Work out the finished part from the listing and answer in its coordinate system (mm). A direction names the side the tool comes from. Coordinates: 2 decimals unless noted, no trailing zeros. Loops run counter-clockwise (first coordinate to the right, second up) from the corner with the lowest first, then second, coordinate; pieces in that order, holes last. Notation, with made-up numbers: M 26.5,-19.5 L 68.5,-19.5 A19 ccw 68.5,-3.5 Z; hole C 42,81 d6. An arc over 180 degrees is marked long. Write each question's results on one line, items separated by ' | '.
```python
from build123d import *

# Parameters (mm, degrees)
SKETCH1_R           = 10.25
BOSS_EXTRUDE1_DEPTH = 2
SKETCH2_R           = 3.4
SKETCH2_R_2         = 2.9
BOSS_EXTRUDE2_DEPTH = 1
SKETCH3_R           = 1.35
CUT_EXTRUDE1_DEPTH  = 15.633010627
SKETCH4_R           = 0.7
CUT_EXTRUDE2_DEPTH  = 15.633010627
CIRPATTERN1_COUNT   = 4
SKETCH5_R           = 4.85
SKETCH5_R_2         = 2.7
BOSS_EXTRUDE3_DEPTH = 3


with BuildPart() as part:
    # Sketch1 → Boss-Extrude1 (new body)
    with BuildSketch(Plane.XY):
        Circle(SKETCH1_R)
    extrude(amount=BOSS_EXTRUDE1_DEPTH)

    # Sketch2 → Boss-Extrude2 (add)
    with BuildSketch(Plane.XY.offset(2)):
        Circle(SKETCH2_R)
        Circle(SKETCH2_R_2, mode=Mode.SUBTRACT)
    extrude(amount=BOSS_EXTRUDE2_DEPTH)

    # Sketch3 → Cut-Extrude1 (cut, through all)
    with BuildSketch(Plane.XY.offset(2)):
        Circle(SKETCH3_R)
    extrude(amount=-CUT_EXTRUDE1_DEPTH, mode=Mode.SUBTRACT)

    # Sketch4 → Cut-Extrude2 (cut, through all)
    with BuildSketch(Plane.XY.offset(2)):
        with Locations((0, 7.25)):
            Circle(SKETCH4_R)
        with Locations((3.5, 7.25)):
            Circle(SKETCH4_R)
        with Locations(Location((-3.5, 7.25, 0), (0, 0, 180))):
            Circle(SKETCH4_R)
        with Locations((-3.5, -7.25)):
            Circle(SKETCH4_R)
        with Locations(Location((3.5, -7.25, 0), (0, 0, 180))):
            Circle(SKETCH4_R)
        with Locations(Location((0, -7.25, 0), (0, 0, 180))):
            Circle(SKETCH4_R)
    cut_extrude2 = extrude(amount=-CUT_EXTRUDE2_DEPTH, mode=Mode.SUBTRACT)

    # CirPattern1: Cut-Extrude2 ×4 about axis
    cirpattern1_axis = Axis((0, 0, 0), (0, 0, 1))
    for i in range(1, CIRPATTERN1_COUNT):
        add(cut_extrude2.rotate(cirpattern1_axis, i * 360 / CIRPATTERN1_COUNT), mode=Mode.SUBTRACT)

    # Sketch5 → Boss-Extrude3 (add)
    with BuildSketch(Plane(origin=(0, 0, 0), x_dir=(-1, 0, 0), z_dir=(0, 0, -1))):
        with Locations(Location((0, 0, 0), (0, 0, 180))):
            Circle(SKETCH5_R)
        Circle(SKETCH5_R_2, mode=Mode.SUBTRACT)
    extrude(amount=BOSS_EXTRUDE3_DEPTH)


solid = part.part
```
1) Find section C-C, the plane y = -7.25. Give the vertices of the cut face in (x, z).
Check result:
outline: M -7.25,0 L -4.2,0 L -4.2,2 L -7.25,2 Z; M -2.8,0 L -0.7,0 L -0.7,2 L -2.8,2 Z; M 0.7,0 L 2.8,0 L 2.8,2 L 0.7,2 Z; M 4.2,0 L 7.25,0 L 7.25,2 L 4.2,2 Z
2) For a pull along Y with two mould halves and no side action, classify faces 4 (the face through (-2.222, -10.006, 0.986)), 5 (the face through (3, 1, 3)), 6 (the face through (-7.84, 0.38, 1.01)) as released by +Y, released by -Y, zero draft, split by the parting line, or undercut.
Check result:
face 4: split by the parting line | face 5: zero draft | face 6: undercut
3) Find section D-D, the plane y = 3.75. Give the vertices of the cut face in (x, z).
Check result:
outline: M -9.54,0 L -7.9,0 L -7.9,2 L -9.54,2 Z; M -6.6,0 L -3.08,0 L -3.08,-3 L 3.08,-3 L 3.08,0 L 6.6,0 L 6.6,2 L -6.6,2 Z; M 7.9,0 L 9.54,0 L 9.54,2 L 7.9,2 Z
4) Find section A-A, the plane x = 0. Give the number of separate pieces and of enclosed holes in the cut face, and give its area (3 significant figures).
Check result:
separate pieces: 4 | enclosed holes: 0 | area: 43.9 mm^2
5) Straight lines are drawn through the part: probe 1 along Y at (x, z) = (0, 1.35); probe 2 along X at (y, z) = (-6.75, 0.9); probe 3 along X at (y, z) = (-3.5, 0.7). For each, find the intervals that lie inside material, in ascending order. Write a range as [from, to].
Check result:
probe 1: [-10.25, -7.95], [-6.55, -1.35], [1.35, 6.55], [7.95, 10.25] | probe 2: [-7.71, -3.99], [-3.01, -0.49], [0.49, 3.01], [3.99, 7.71] | probe 3: [-9.63, -7.95], [-6.55, 6.55], [7.95, 9.63]
6) Given pin 1 Ø5 at (x, y) = (2, 6.5) entering from +Z; pin 2 Ø3 at (x, y) = (8, -1) entering from -Z, each flat-ended and moving along its own axis, determine where each tip first touches the part or whether it passes through.
Check result:
pin 1: z = 2 | pin 2: z = 0
7) Which of the six approach directions +Z, -Z, +X, -X, +Y, -Y give full straight-line access (tool end or side, diameter ignored) to faces 1 (the face through (-1.051, 4.735, -1.479)), 2 (the face through (-2.9, 0.1, 2.5)), 3 (the face through (-7.944, 3.409, 1.014))?
Check result:
face 1: -Z | face 2: +Z | face 3: +Z, -Z
